from build123d import *

# Parameters (mm, degrees)
F0_W     = 20
F0_H     = 20
F0_W_2   = 16.8
F0_H_2   = 16.8
F1_DEPTH = 351.5
F2_R     = 5.25
F3_DEPTH = 5


# Not quite as in the source:
# - a feature names something its author has since deleted; it is built from what else it names


with BuildPart() as f1:
    # F0 (on Front) → F1 (new body)
    with BuildSketch(Plane.XZ):
        with Locations((10, -10)):
            Rectangle(F0_W, F0_H)
        with Locations((10, -10)):
            Rectangle(F0_W_2, F0_H_2, mode=Mode.SUBTRACT)
    extrude(amount=F1_DEPTH)

    # F2 (on face) → F3 (cut)
    with BuildSketch(Plane.XY):
        with Locations((10, -310.75)):
            Circle(F2_R)
        with Locations((10, -283.75)):
            Circle(F2_R)
        with Locations((10, -256.75)):
            Circle(F2_R)
        with Locations((10, -229.75)):
            Circle(F2_R)
        with Locations((10, -202.75)):
            Circle(F2_R)
        with Locations((10, -175.75)):
            Circle(F2_R)
        with Locations((10, -148.75)):
            Circle(F2_R)
        with Locations((10, -121.75)):
            Circle(F2_R)
        with Locations((10, -94.75)):
            Circle(F2_R)
        with Locations((10, -67.75)):
            Circle(F2_R)
        with Locations((10, -40.75)):
            Circle(F2_R)
        with Locations((10, -13.75)):
            Circle(F2_R)
        with Locations((10, -337.75)):
            Circle(F2_R)
    extrude(amount=-F3_DEPTH, mode=Mode.SUBTRACT)


solid = f1.part
Input: part model. Units: mm. Frame: model coordinates. A direction names the side the tool comes from. Give positions to 0.01 mm unless a question says otherwise; leave off trailing zeros. Write each loop counter-clockwise with the first axis right and the second up, starting at its lowest first coordinate (ties: lowest second). Pieces come first, ordered by that corner, then holes. Notation, with made-up numbers: M 36.5,-13 L 89.5,-13 A12 cw 89.5,-3 Z; hole C 80.25,26.5 d8. An arc over 180 degrees is marked long. Use one line per item in the form item = value.
1. Cut plane B-B on y = -67.75. Return loops of the section in (x, z), and give its area (3 significant figures).
Outcome:
outline = M 0,-20 L 20,-20 L 20,0 L 15.25,0 L 15.25,-1.6 L 18.4,-1.6 L 18.4,-18.4 L 1.6,-18.4 L 1.6,-1.6 L 4.75,-1.6 L 4.75,0 L 0,0 Z
area = 101 mm²
2. Mould query, pull axis X, two halves, no side actions, for faces 4 (the face through (0, -173, -10)), 5 (the face through (4, -173, -1.6)), 6 (the face through (10, -351.5, -19)), 7 (the face through (8.862, -153.875, -0.789)). Classes: released by +X, released by -X, zero draft, split by the parting line, or undercut.
Outcome:
face_4 = released by -X
face_5 = undercut
face_6 = zero draft
face_7 = undercut
3. Cut plane D-D on x = 10.25. State how many separate pieces and enclosed holes the cut face has, and give its area (3 significant figures).
Outcome:
separate_pieces = 15
enclosed_holes = 0
area = 907 mm²
4. Cut plane C-C on y = -215. Return loops of the section in (x, z).
Outcome:
outline = M 0,-20 L 20,-20 L 20,0 L 0,0 Z; hole M 1.6,-18.4 L 18.4,-18.4 L 18.4,-1.6 L 1.6,-1.6 Z
5. Reachability of faces 1 (the face through (1.6, -173, -10)), 2 (the face through (20, -173, -10)), 3 (the face through (12.82, -306.32, -0.79)) from +Z, -Z, +X, -X, +Y, -Y: full face, straight path, thin tool, end or side. Return the list, or none.
Outcome:
face_1 = +Y, -Y
face_2 = +Z, -Z, +X, +Y, -Y
face_3 = +Z
6. Cut plane A-A on z = -6.75. Return loops of the section in (x, y).
Outcome:
outline = M 0,-351.5 L 1.6,-351.5 L 1.6,0 L 0,0 Z; M 18.4,-351.5 L 20,-351.5 L 20,0 L 18.4,0 Z
7. First-contact query: P1, Ø9.5, axis at x = 10, y = -67.75, coming from the +Z side; P2, Ø4, axis at x = 16, z = -3, coming from the -Y side. Flat tips, straight axial feed; report the tip coordinate or a pass-through.
Outcome:
P1 = -18.4
P2 = -351.5
8. Ray query, L1, parallel to X at y = -125, z = -16.5; L2, parallel to Z at x = 2.5, y = -230; L3, parallel to Z at x = 7.5, y = -90.5. Return the intervals inside material, ascending.
Outcome:
L1 = 0 to 1.6, 18.4 to 20
L2 = -20 to -18.4, -1.6 to 0
L3 = -20 to -18.4
